```python
from build123d import *

# Parameters (mm, degrees)
SKETCH1_W                       = 75
SKETCH1_H                       = 50
BOSS_EXTRUDE1_DEPTH             = 1
BOSS_EXTRUDE2_REACH             = 43.356
SKETCH2_W                       = 45
SKETCH2_H                       = 10
BOSS_EXTRUDE2_DIRECTION_2_REACH = 10.644
BOSS_EXTRUDE5_DEPTH             = 33


with BuildPart() as part:
    # Sketch1 → Boss-Extrude1 (new body)
    with BuildSketch(Plane.XY):
        with Locations((-4.920212766, 16.356382979)):
            Rectangle(SKETCH1_W, SKETCH1_H)
    extrude(amount=BOSS_EXTRUDE1_DEPTH)

    # Boss-Extrude2: up to this face of the body (flat: up to its plane)
    boss_extrude2_end = Plane(part.part.faces().sort_by_distance((-4.920212766, 41.356382979, 0.5))[0])
    # Sketch2 → Boss-Extrude2 (add, up to the picked face)
    with BuildSketch(Plane(origin=(0, 0, 0), x_dir=(1, 0, 0), z_dir=(0, 1, 0)), mode=Mode.PRIVATE) as boss_extrude2_sk1:
        with Locations((-4.920212766, -6)):
            Rectangle(SKETCH2_W, SKETCH2_H)
    boss_extrude2_tool1 = split(extrude(boss_extrude2_sk1.sketch, amount=BOSS_EXTRUDE2_REACH, mode=Mode.PRIVATE), bisect_by=boss_extrude2_end, keep=Keep.BOTH, mode=Mode.PRIVATE)
    add(boss_extrude2_tool1.solids().sort_by_distance((-4.920213, 0, 6))[0])

    # Boss-Extrude2 direction 2: up to this face of the body (flat: up to its plane)
    boss_extrude2_direction_2_end = Plane(part.part.faces().sort_by_distance((-4.920212766, -8.643617021, 0.5))[0])
    # Sketch2 → Boss-Extrude2 direction 2 (add, up to the picked face)
    with BuildSketch(Plane(origin=(0, 0, 0), x_dir=(1, 0, 0), z_dir=(0, 1, 0)), mode=Mode.PRIVATE) as boss_extrude2_direction_2_sk1:
        with Locations((-4.920212766, -6)):
            Rectangle(SKETCH2_W, SKETCH2_H)
    boss_extrude2_direction_2_tool1 = split(extrude(boss_extrude2_direction_2_sk1.sketch, amount=-BOSS_EXTRUDE2_DIRECTION_2_REACH, mode=Mode.PRIVATE), bisect_by=boss_extrude2_direction_2_end, keep=Keep.BOTH, mode=Mode.PRIVATE)
    add(boss_extrude2_direction_2_tool1.solids().sort_by_distance((-4.920213, 0, 6))[0])

    # Sketch4 → Boss-Extrude5 (add)
    with BuildSketch(Plane(origin=(0, 0, 0), x_dir=(1, 0, 0), z_dir=(0, 1, 0))):
        Polygon((-40.49649997, 0), (-36.49649997, 14), (-31.49649997, 14), (-31.49649997, 0), align=None)
        Polygon((21.656074438, 0), (30.656074438, 0), (26.656074438, 14), (21.656074438, 14), align=None)
    extrude(amount=BOSS_EXTRUDE5_DEPTH)


solid = part.part
```
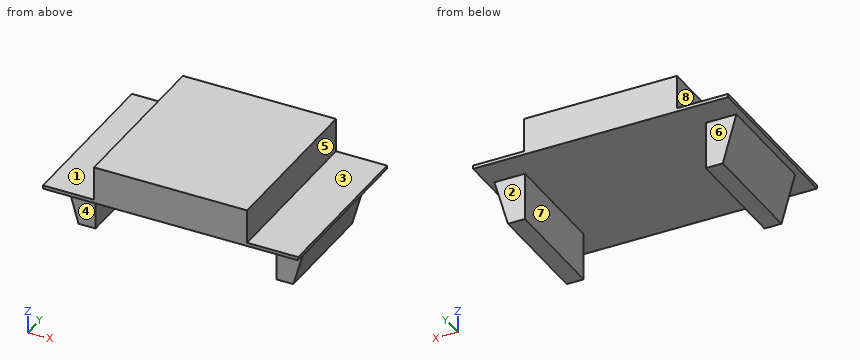
Geometry check sheet. Reference: the model listing, model coordinates, mm. Face numbers are marked on the shaded views. A direction names the side the tool comes from. Coordinates: 2 decimals unless noted, no trailing zeros. Order: outer loops, then holes, each group sorted by start corner. A loop starts at its lowest first (then second) coordinate and runs counter-clockwise, first axis right, second up.
Q1. Sectioned sample at D-D on z = 3.5. Record the cut outline in (x, y).
Reply:
outline: (-27.42, -8.64) - (17.58, -8.64) - (17.58, 41.36) - (-27.42, 41.36) - close
Q2. Sectioned sample at B-B on x = -33. Record the cut outline in (y, z), and give its area (3 significant figures).
Reply:
outline: (-8.64, 0) - (0, 0) - (0, -14) - (33, -14) - (33, 0) - (41.36, 0) - (41.36, 1) - (-8.64, 1) - close
area: 512 mm2
Q3. Thickness scan on probe 1 along Z at (x, y) = (22, 29); probe 2 along Z at (x, y) = (-25.5, -3); probe 3 along X at (y, z) = (16, -3.75). Record the ranges inside material, lowest first.
Reply:
probe 1: z = -14 to 1
probe 2: z = 0 to 11
probe 3: x = -39.43 to -31.5, 21.66 to 29.58
Q4. Sectioned sample at A-A on z = -10.75. Record the cut outline in (x, y).
Reply:
outline: (-37.43, 0) - (-31.5, 0) - (-31.5, 33) - (-37.43, 33) - close; (21.66, 0) - (27.58, 0) - (27.58, 33) - (21.66, 33) - close
Q5. Sectioned sample at C-C on y = 23.5. Record the cut outline in (x, z), and give its area (3 significant figures).
Reply:
outline: (-42.42, 0) - (-40.5, 0) - (-36.5, -14) - (-31.5, -14) - (-31.5, 0) - (21.66, 0) - (21.66, -14) - (26.66, -14) - (30.66, 0) - (32.58, 0) - (32.58, 1) - (17.58, 1) - (17.58, 11) - (-27.42, 11) - (-27.42, 1) - (-42.42, 1) - close
area: 721 mm2
Q6. Tool access check on the marked faces 1, 2, 3 and 4. Record the directions out of +Z, -Z, +X, -X, +Y, -Y that give a thin tool (end or side, any length) a straight path to the whole face; none if there is none.
Reply:
face 1: +Z, -X, +Y, -Y
face 2: -Z, +X, -X, +Y
face 3: +Z, +X, +Y, -Y
face 4: -Z, +X, -X, -Y
Q7. Draft check along X on the marked faces 5, 6, 7 and 8. Enter one of: released by +X, released by -X, zero draft, split by the parting line, or undercut.
Reply:
face 5: released by +X
face 6: zero draft
face 7: undercut
face 8: released by -X
Q8. Depth check by flat-ended pin: pin 1 Ø4.5 at (x, y) = (27.5, 25.5) entering from +Z; pin 2 Ø7 at (x, z) = (26, -10.5) entering from -Y; pin 3 Ø4 at (y, z) = (21.5, -4) entering from +X. Enter the tip coordinate at first touch or a pass-through.
Reply:
pin 1: stops at z = 1
pin 2: stops at y = 0
pin 3: stops at x = 30.08
